Input: part model. Units: mm. Frame: model coordinates. A direction names the side the tool comes from. Round coordinates to 2 decimals unless told otherwise and drop trailing zeros. Write each loop counter-clockwise with the first axis right and the second up, starting at its lowest first coordinate (ties: lowest second). Pieces come first, ordered by that corner, then holes. Notation, with made-up numbers: (86, -30.75) - (93, -30.75) arc R21 cw to (93, -16.75) - close; hole circle Ø7 at (0.5, 69.5). An arc over 180 degrees is marked (long way). Use one line per item in the form item = value.
```python
from build123d import *

# Parameters (mm, degrees)
SKETCH1_W               = 39.6
SKETCH1_H               = 39.6
BOSS_EXTRUDE1_DEPTH     = 25
CUT_EXTRUDE1_DEPTH      = 5
CUT_EXTRUDE2_DEPTH      = 38.537714368
CUT_EXTRUDE2_DEPTH_BACK = 38.537714368
SKETCH3_R               = 2.75
CUT_EXTRUDE4_START      = 25
CUT_EXTRUDE4_DEPTH      = 5


with BuildPart() as part:
    # Sketch1 → Boss-Extrude1 (new body)
    with BuildSketch(Plane(origin=(0, 0, 0), x_dir=(0, 0, -1), z_dir=(1, 0, 0))):
        Rectangle(SKETCH1_W, SKETCH1_H)
    extrude(amount=BOSS_EXTRUDE1_DEPTH)

    # Sketch2 → Cut-Extrude1 (cut)
    with BuildSketch(Plane(origin=(0, 0, 0), x_dir=(0, 0, -1), z_dir=(1, 0, 0))):
        Polygon((4.67653718, 0), (2.33826859, 4.05), (-2.33826859, 4.05), (-4.67653718, 0), (-2.33826859, -4.05), (2.33826859, -4.05), align=None)
    extrude(amount=CUT_EXTRUDE1_DEPTH, mode=Mode.SUBTRACT)

    # Sketch3 → Cut-Extrude2 (cut, two sides: drawn at the far end of the back side and taken through both)
    with BuildSketch(Plane(origin=(0, 0, 0), x_dir=(0, 0, -1), z_dir=(1, 0, 0)).offset(-CUT_EXTRUDE2_DEPTH_BACK)):
        Circle(SKETCH3_R)
    extrude(amount=CUT_EXTRUDE2_DEPTH + CUT_EXTRUDE2_DEPTH_BACK, mode=Mode.SUBTRACT)

    # Sketch2<2> → Cut-Extrude4 (cut)
    with BuildSketch(Plane(origin=(0, 0, 0), x_dir=(0, 0, -1), z_dir=(1, 0, 0)).offset(CUT_EXTRUDE4_START)):
        Polygon((4.67653718, 0), (2.33826859, 4.05), (-2.33826859, 4.05), (-4.67653718, 0), (-2.33826859, -4.05), (2.33826859, -4.05), align=None)
    extrude(amount=-CUT_EXTRUDE4_DEPTH, mode=Mode.SUBTRACT)


solid = part.part
```
(1) Material intervals for L1, parallel to Z at x = 16, y = 0; L2, parallel to Y at x = 4, z = -1.5, sorted ascending.
Derived:
L1 = -19.8 to -2.75, 2.75 to 19.8
L2 = -19.8 to -4.05, 4.05 to 19.8
(2) Cut plane A-A on z = 0. Output: boundary loops of the cut face in (x, y).
Derived:
outline = (0, -19.8) - (25, -19.8) - (25, -4.05) - (20, -4.05) - (20, -2.75) - (5, -2.75) - (5, -4.05) - (0, -4.05) - close; (0, 4.05) - (5, 4.05) - (5, 2.75) - (20, 2.75) - (20, 4.05) - (25, 4.05) - (25, 19.8) - (0, 19.8) - close
(3) Cut plane B-B on x = 10.75. Output: boundary loops of the cut face in (y, z), then the cut area to 3 significant figures.
Derived:
outline = (-19.8, -19.8) - (19.8, -19.8) - (19.8, 19.8) - (-19.8, 19.8) - close; hole circle Ø5.5 at (0, 0)
area = 1,540 mm^2
(4) Access query for faces 1 (the face through (12, 0, -19.8)), 2 (the face through (23, 4.05, 0)), 3 (the face through (2.46, -2, 3.52)). Directions: +Z, -Z, +X, -X, +Y, -Y. A direction counts if a zero-diameter tool reaches every point of the face in a straight line with its end or side. Return the directions, or none.
Derived:
face_1 = -Z, +X, -X, +Y, -Y
face_2 = +X
face_3 = -X
(5) Draft query along Y for faces 4 (the face through (2.46, 2, -3.52)), 5 (the face through (0, 0, 5)), 6 (the face through (12, 19.8, 0)). Return one class per face: released by +Y, released by -Y, zero draft, split by the parting line, or undercut.
Derived:
face_4 = undercut
face_5 = zero draft
face_6 = released by +Y
(6) Cut plane C-C on x = 23.75. Output: boundary loops of the cut face in (y, z).
Derived:
outline = (-19.8, -19.8) - (19.8, -19.8) - (19.8, 19.8) - (-19.8, 19.8) - close; hole (-4.05, -2.34) - (0, -4.68) - (4.05, -2.34) - (4.05, 2.34) - (0, 4.68) - (-4.05, 2.34) - close
